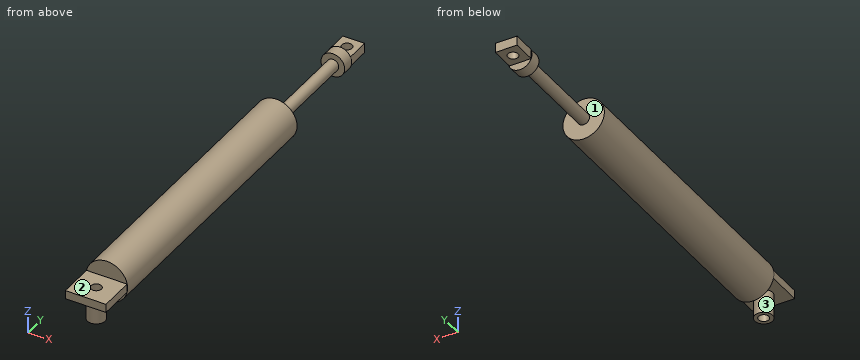
from build123d import *

# Parameters (mm, degrees)
SKETCH1_R           = 11.1125
BOSS_EXTRUDE1_DEPTH = 152.4
SKETCH2_R           = 3.175
BOSS_EXTRUDE2_DEPTH = 50.8
SKETCH3_W           = 21.757515496
SKETCH3_H           = 4.530998995
BOSS_EXTRUDE3_DEPTH = 19.05
SKETCH4_R           = 2.778125
CUT_EXTRUDE1_DEPTH  = 19.05
SKETCH5_R           = 4.7625
SKETCH5_R_2         = 2.778125
BOSS_EXTRUDE4_DEPTH = 12.7
SKETCH6_R           = 6.35
BOSS_EXTRUDE5_DEPTH = 6.35
SKETCH7_W           = 11.625186508
SKETCH7_H           = 5.08
BOSS_EXTRUDE6_DEPTH = 12.7
SKETCH8_R           = 2.778125
CUT_EXTRUDE2_DEPTH  = 12.7


with BuildPart() as part:
    # Sketch1 → Boss-Extrude1 (new body)
    with BuildSketch(Plane(origin=(0, 0, 0), x_dir=(1, 0, 0), z_dir=(0, 1, 0))):
        with Locations(Location((0, 0, 0), (0, 0, 90))):
            Circle(SKETCH1_R)
    extrude(amount=BOSS_EXTRUDE1_DEPTH)

    # Sketch2 → Boss-Extrude2 (add)
    with BuildSketch(Plane(origin=(0, 152.4, 0), x_dir=(1, 0, 0), z_dir=(0, 1, 0))):
        with Locations(Location((0, 0, 0), (0, 0, 270))):
            Circle(SKETCH2_R)
    extrude(amount=BOSS_EXTRUDE2_DEPTH)

    # Sketch3 → Boss-Extrude3 (add)
    with BuildSketch(Plane.XZ):
        with Locations((-0.018003691, -0.086452367)):
            Rectangle(SKETCH3_W, SKETCH3_H)
    extrude(amount=BOSS_EXTRUDE3_DEPTH)

    # Sketch4 → Cut-Extrude1 (cut)
    with BuildSketch(Plane.XY.offset(2.179047131)):
        with Locations((0, -9.525)):
            Circle(SKETCH4_R)
    extrude(amount=-CUT_EXTRUDE1_DEPTH, mode=Mode.SUBTRACT)

    # Sketch5 → Boss-Extrude4 (add)
    with BuildSketch(Plane(origin=(0, 0, -2.351951864), x_dir=(-1, 0, 0), z_dir=(0, 0, -1))):
        with Locations(Location((0, -9.525, 0), (0, 0, 180))):
            Circle(SKETCH5_R)
        with Locations(Location((0, -9.525, 0), (0, 0, 180))):
            Circle(SKETCH5_R_2, mode=Mode.SUBTRACT)
    extrude(amount=BOSS_EXTRUDE4_DEPTH)

    # Sketch6 → Boss-Extrude5 (add)
    with BuildSketch(Plane(origin=(0, 203.2, 0), x_dir=(1, 0, 0), z_dir=(0, 1, 0))):
        with Locations(Location((0, 0, 0), (0, 0, 270))):
            Circle(SKETCH6_R)
    extrude(amount=BOSS_EXTRUDE5_DEPTH)

    # Sketch7 → Boss-Extrude6 (add)
    with BuildSketch(Plane(origin=(0, 209.55, 0), x_dir=(1, 0, 0), z_dir=(0, 1, 0))):
        with Locations((-0.116507708, -0.266618865)):
            Rectangle(SKETCH7_W, SKETCH7_H)
    extrude(amount=BOSS_EXTRUDE6_DEPTH)

    # Sketch8 → Cut-Extrude2 (cut)
    with BuildSketch(Plane.XY.offset(2.806618865)):
        with Locations((0, 215.9)):
            Circle(SKETCH8_R)
    extrude(amount=-CUT_EXTRUDE2_DEPTH, mode=Mode.SUBTRACT)


solid = part.part
For this review, take the finished solid that the model builds, in its own axes (mm). Face numbers are marked on the shaded views. A direction names the side the tool comes from. Coordinates: 2 decimals unless noted, no trailing zeros. Loops run counter-clockwise (first coordinate to the right, second up) from the corner with the lowest first, then second, coordinate; pieces in that order, holes last. Notation, with made-up numbers: (80, -6) - (135, -6) arc R22 cw to (135, 24) - close; hole circle Ø5 at (22, 57.5). An arc over 180 degrees is marked (long way). Use a Markdown table: item, result. Add a question column.
Item 1: We need section B-B (y = 215.9). Give the boundary of the cut face in (x, z).
Item 2: Tool access review of the marked faces 1, 2 and 3: name each direction out of +Z, -Z, +X, -X, +Y, -Y from which nothing blocks a thin tool from reaching the whole face with its end or side.
Item 3: We need section D-D (y = 96). Give the boundary of the cut face in (x, z) (1 decimal), and give its area (3 significant figures).
Item 4: We need section A-A (x = 0). Give the number of separate pieces and of enclosed holes in the cut face, and give its area (3 significant figures).
Item 5: For line 1 (Y direction, x = 0, z = -0.25); line 2 (X direction, y = 215.9, z = 1.4); line 3 (Y direction, x = 2, z = -2.5), list the stretches that pass through material, from the lowest coordinate up.
Item 6: Insertion check: pin 1 Ø5 at (x, z) = (-7, -7) entering from +Y; pin 2 Ø3 at (y, z) = (68, -2.5) entering from -X; pin 3 Ø2 at (x, z) = (-0.5, 6) entering from -Y. Each pin has a flat end and moves straight along its axis. Give the tip position at first contact, or say it passes through.
Results list:
| question | item | result |
|---|---|---|
| 1 | outline | (-5.93, -2.27) - (-2.78, -2.27) - (-2.78, 2.81) - (-5.93, 2.81) - close; (2.78, -2.27) - (5.7, -2.27) - (5.7, 2.81) - (2.78, 2.81) - close |
| 2 | face 1 | none |
| 2 | face 2 | +Z, +X, -X, -Y |
| 2 | face 3 | -Z |
| 3 | outline | circle Ø22.2 at (0, 0) |
| 3 | area | 388 mm^2 |
| 4 | separate pieces | 3 |
| 4 | enclosed holes | 0 |
| 4 | area | 3,940 mm^2 |
| 5 | line 1 | y = -19.05 to -12.3, -6.75 to 213.12, 218.68 to 222.25 |
| 5 | line 2 | x = -5.93 to -2.78, 2.78 to 5.7 |
| 5 | line 3 | y = -13.85 to -11.45, -7.6 to -5.2, 0 to 152.4, 203.2 to 209.55 |
| 6 | pin 1 | stops at y = 152.4 |
| 6 | pin 2 | stops at x = -11.07 |
| 6 | pin 3 | stops at y = 0 |
